from build123d import *

# Parameters (mm, degrees)
SKETCH1_W                                        = 76.2
SKETCH1_H                                        = 76.2
BOSS_EXTRUDE1_DEPTH                              = 19.05
CBORE_FOR_1_2_SOCKET_HEAD_CAP_SCREW1_D           = 13.49248
CBORE_FOR_1_2_SOCKET_HEAD_CAP_SCREW1_CBORE_D     = 20.6375
CBORE_FOR_1_2_SOCKET_HEAD_CAP_SCREW1_CBORE_DEPTH = 12.7


with BuildPart() as part:
    # Sketch1 → Boss-Extrude1 (new body)
    with BuildSketch(Plane(origin=(0, 0, 0), x_dir=(1, 0, 0), z_dir=(0, 1, 0))):
        with Locations((38.1, 38.1)):
            Rectangle(SKETCH1_W, SKETCH1_H)
    extrude(amount=BOSS_EXTRUDE1_DEPTH)

    # CBORE for 1/2 Socket Head Cap Screw1 (through all)
    with Locations(Plane(origin=(0, 19.05, 0), x_dir=(1, 0, 0), z_dir=(0, 1, 0))):
        with Locations((57.15, 57.15)):
            CounterBoreHole(CBORE_FOR_1_2_SOCKET_HEAD_CAP_SCREW1_D / 2, CBORE_FOR_1_2_SOCKET_HEAD_CAP_SCREW1_CBORE_D / 2, CBORE_FOR_1_2_SOCKET_HEAD_CAP_SCREW1_CBORE_DEPTH)

    # Mirror1: part across plane


with BuildPart() as part_1:
    add(part.part)
    add(part.part.mirror(Plane(origin=(0, 19.05, 0), x_dir=(1, 0, 0), z_dir=(0, 0, -1))))

    # Mirror2: part across plane


with BuildPart() as part_2:
    add(part_1.part)
    add(part_1.part.mirror(Plane(origin=(0, 19.05, 0), x_dir=(0, 0, 1), z_dir=(1, 0, 0))))


solid = part_2.part
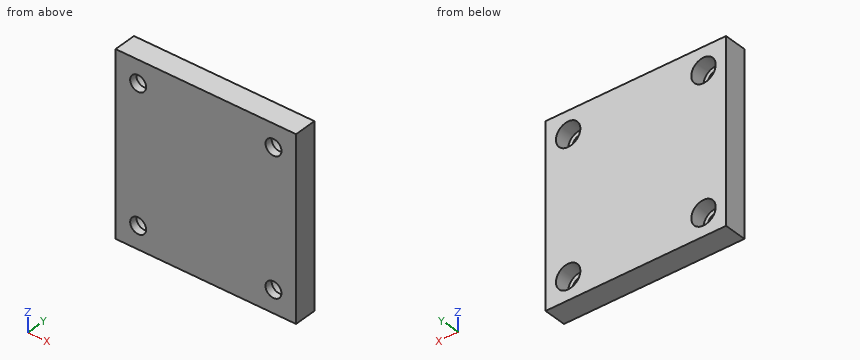
For this review, take the finished solid that the model builds, in its own axes (mm). Round coordinates to 2 decimals unless told otherwise and drop trailing zeros. Loops run counter-clockwise (first coordinate to the right, second up) from the corner with the lowest first, then second, coordinate; pieces in that order, holes last. Notation, with made-up numbers: (9.5, 55.5) - (36.5, 55.5) arc R9 ccw to (36.5, 61.5) - close; hole circle Ø2 at (49, 76). An arc over 180 degrees is marked (long way). One line per question, with ' | ' between items.
Q1. Take a section at A-A (x = -57.15). Give the boundary of the cut face in (y, z).
Taken from the geometry:
outline: (0, -76.2) - (19.05, -76.2) - (19.05, -67.47) - (6.35, -67.47) - (6.35, -63.9) - (0, -63.9) - close; (0, -50.4) - (6.35, -50.4) - (6.35, -46.83) - (19.05, -46.83) - (19.05, 46.83) - (6.35, 46.83) - (6.35, 50.4) - (0, 50.4) - close; (0, 63.9) - (6.35, 63.9) - (6.35, 67.47) - (19.05, 67.47) - (19.05, 76.2) - (0, 76.2) - close
Q2. Take a section at B-B (y = 16.5). Give the boundary of the cut face in (x, z), and give its area (3 significant figures).
Taken from the geometry:
outline: (-76.2, -76.2) - (76.2, -76.2) - (76.2, 76.2) - (-76.2, 76.2) - close; hole circle Ø20.64 at (-57.15, -57.15); hole circle Ø20.64 at (-57.15, 57.15); hole circle Ø20.64 at (57.15, -57.15); hole circle Ø20.64 at (57.15, 57.15) | area: 21,900 mm²
Q3. Take a section at C-C (z = 57.15). Give the boundary of the cut face in (x, y), and give its area (3 significant figures).
Taken from the geometry:
outline: (-76.2, 0) - (-63.9, 0) - (-63.9, 6.35) - (-67.47, 6.35) - (-67.47, 19.05) - (-76.2, 19.05) - close; (-50.4, 0) - (50.4, 0) - (50.4, 6.35) - (46.83, 6.35) - (46.83, 19.05) - (-46.83, 19.05) - (-46.83, 6.35) - (-50.4, 6.35) - close; (63.9, 0) - (76.2, 0) - (76.2, 19.05) - (67.47, 19.05) - (67.47, 6.35) - (63.9, 6.35) - close | area: 2,210 mm²
Q4. For pin 1 (16.5 mm diameter, centred on x = -58.5, z = 57.5, fed in from +Y), flat-tipped, find the tip position at first contact; note if it passes through.
Taken from the geometry:
pin 1: stops at y = 6.35
Q5. For line 1 along Z through (x, y) = (-57.15, 4); line 2 along Z through (x, y) = (-57.15, 15.25), list the stretches that pass through material, from the lowest coordinate up. Write a range as [from, to].
Taken from the geometry:
line 1: z = [-76.2, -63.9], [-50.4, 50.4], [63.9, 76.2] | line 2: z = [-76.2, -67.47], [-46.83, 46.83], [67.47, 76.2]
